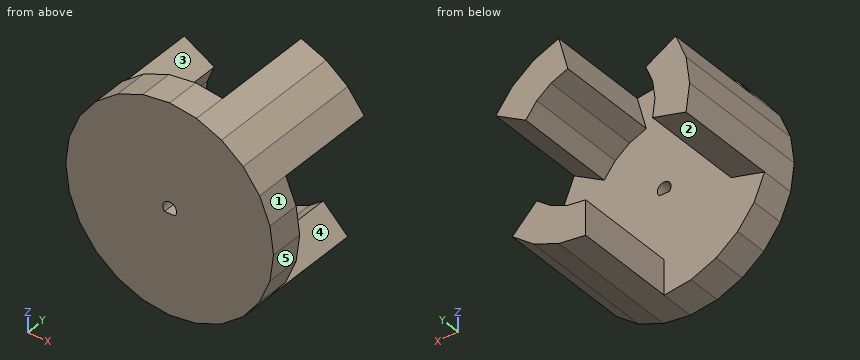
```python
from build123d import *

# Parameters (mm, degrees)
BOSS_EXTRUDE3_DEPTH   = 40
BOSS_EXTRUDE3_2_DEPTH = 40
BOSS_EXTRUDE3_3_DEPTH = 40
BOSS_EXTRUDE4_DEPTH   = 10


with BuildPart() as part:
    # Sketch1 → Boss-Extrude3 (new body)
    with BuildSketch(Plane(origin=(0, 0, 0), x_dir=(1, 0, 0), z_dir=(0, 1, 0))):
        Polygon((14.264167555, 14.264167555), (10.086289606, 17.469966057), (5.221047689, 19.485215243), (0, 20.172579212), (0, 30.258868817), (7.831571533, 29.227822865), (15.129434409, 26.204949086), (21.396251332, 21.396251332), align=None)
    extrude(amount=BOSS_EXTRUDE3_DEPTH)



with BuildPart() as body_2:
    # Sketch1 → Boss-Extrude3 2 (new body)
    with BuildSketch(Plane(origin=(0, 0, 0), x_dir=(1, 0, 0), z_dir=(0, 1, 0))):
        Polygon((5.221047689, -19.485215243), (10.086289606, -17.469966057), (14.264167555, -14.264167555), (17.469966057, -10.086289606), (26.204949086, -15.129434409), (21.396251332, -21.396251332), (15.129434409, -26.204949086), (7.831571533, -29.227822865), align=None)
    extrude(amount=BOSS_EXTRUDE3_2_DEPTH)


with BuildPart() as body_3:
    # Sketch1 → Boss-Extrude3 3 (new body)
    with BuildSketch(Plane(origin=(0, 0, 0), x_dir=(1, 0, 0), z_dir=(0, 1, 0))):
        Polygon((-19.485215243, 5.221047689), (-20.172579212, 0), (-19.485215243, -5.221047689), (-17.469966057, -10.086289606), (-26.204949086, -15.129434409), (-29.227822865, -7.831571533), (-30.258868817, 0), (-29.227822865, 7.831571533), align=None)
    extrude(amount=BOSS_EXTRUDE3_3_DEPTH)


with BuildPart() as part_1:
    add(part.part)

    add(body_2.part)  # Boss-Extrude4 merges body 2

    add(body_3.part)  # Boss-Extrude4 merges body 3
    # Sketch1_6 → Boss-Extrude4 (add)
    with BuildSketch(Plane(origin=(0, 0, 0), x_dir=(1, 0, 0), z_dir=(0, 1, 0))):
        Polygon((-29.227822865, 7.831571533), (-19.485215243, 5.221047689), (-20.172579212, 0), (-19.485215243, -5.221047689), (-17.469966057, -10.086289606), (-26.204949086, -15.129434409), (-21.396251332, -21.396251332), (-15.129434409, -26.204949086), (-7.831571533, -29.227822865), (0, -30.258868817), (7.831571533, -29.227822865), (5.221047689, -19.485215243), (10.086289606, -17.469966057), (14.264167555, -14.264167555), (17.469966057, -10.086289606), (26.204949086, -15.129434409), (29.227822865, -7.831571533), (30.258868817, 0), (29.227822865, 7.831571533), (26.204949086, 15.129434409), (21.396251332, 21.396251332), (14.264167555, 14.264167555), (10.086289606, 17.469966057), (5.221047689, 19.485215243), (0, 20.172579212), (0, 30.258868817), (-7.831571533, 29.227822865), (-15.129434409, 26.204949086), (-21.396251332, 21.396251332), (-26.204949086, 15.129434409), align=None)
        with BuildLine():
            Line((-1.5, 1.322875656), (1.5, 1.322875656))
            ThreePointArc((1.5, 1.322875656), (0, -2), (-1.5, 1.322875656))
        make_face(mode=Mode.SUBTRACT)
    extrude(amount=BOSS_EXTRUDE4_DEPTH)


solid = part_1.part
```
Input: part model. Units: mm. Frame: model coordinates. Face numbers are marked on the shaded views. A direction names the side the tool comes from. Give positions to 0.01 mm unless a question says otherwise; leave off trailing zeros. Order: outer loops, then holes, each group sorted by start corner. A loop starts at its lowest first (then second) coordinate and runs counter-clockwise, first axis right, second up. Notation, with made-up numbers: M -38,-7.5 L 10,-7.5 A14 ccw 10,6.5 Z; hole C 4.25,-19.75 d1. An arc over 180 degrees is marked long. Return JSON: item names as keys, results as strings.
1) Contact query for flat-ended pins moving along their axis: pin 1 (6 mm diameter, centred on x = 21.5, z = 6, fed in from +Y); pin 2 (4 mm diameter, centred on y = 28, z = -23, fed in from +X); pin 3 (5 mm diameter, centred on y = 18.5, z = 11, fed in from +X). Output: stop coordinate, or through.
Taken from the geometry:
{"pin 1": "stops at y = 10", "pin 2": "stops at x = 21.4", "pin 3": "stops at x = 23.38"}
2) Access query for the marked faces 1 and 2. Directions: +Z, -Z, +X, -X, +Y, -Y. A direction counts if a zero-diameter tool reaches every point of the face in a straight line with its end or side. Return the directions, or none.
Taken from the geometry:
{"face 1": "+Z, +X, +Y, -Y", "face 2": "-Z, +X, +Y"}
3) Section query D-D on z = 16. Output: boundary loops of the cut face in (x, y), and give its area (3 significant figures).
Taken from the geometry:
{"outline": "M -25.54,0 L 25.54,0 L 25.54,40 L 12,40 L 12,10 L -25.54,10 Z", "area": "917 mm2"}
4) Section query A-A on y = 22. Output: boundary loops of the cut face in (x, z), and give its area (3 significant figures).
Taken from the geometry:
{"outline": "M -30.26,0 L -29.23,-7.83 L -19.49,-5.22 L -20.17,0 L -19.49,5.22 L -17.47,10.09 L -26.2,15.13 L -29.23,7.83 Z; M 0,-30.26 L 7.83,-29.23 L 15.13,-26.2 L 21.4,-21.4 L 14.26,-14.26 L 10.09,-17.47 L 5.22,-19.49 L 0,-20.17 Z; M 5.22,19.49 L 10.09,17.47 L 14.26,14.26 L 17.47,10.09 L 26.2,15.13 L 21.4,21.4 L 15.13,26.2 L 7.83,29.23 Z", "area": "592 mm2"}
5) Mould query, pull axis Z, two halves, no side actions, for the marked faces 3, 4 and 5. Classes: released by +Z, released by -Z, zero draft, split by the parting line, or undercut.
Taken from the geometry:
{"face 3": "released by +Z", "face 4": "undercut", "face 5": "released by -Z"}
6) Line query: L1, parallel to Z at x = 0, y = 5; L2, parallel to X at y = 5, z = 0; L3, parallel to Y at x = -14.5, z = 20.5. Output: solid intervals per line, ascending. Write a range as [from, to].
Taken from the geometry:
{"L1": "z = [-30.26, -1.32], [2, 30.26]", "L2": "x = [-30.26, -2], [2, 30.26]", "L3": "y = [0, 10]"}
7) Section query C-C on x = 6. Output: boundary loops of the cut face in (y, z), and give its area (3 significant figures).
Taken from the geometry:
{"outline": "M 0,-29.47 L 40,-29.47 L 40,-19.16 L 10,-19.16 L 10,19.16 L 40,19.16 L 40,22.39 L 10,22.39 L 10,29.47 L 0,29.47 Z", "area": "995 mm2"}
8) Section query B-B on y = 9. Output: boundary loops of the cut face in (x, z), and give its area (3 significant figures).
Taken from the geometry:
{"outline": "M -30.26,0 L -29.23,-7.83 L -26.2,-15.13 L -21.4,-21.4 L -15.13,-26.2 L -7.83,-29.23 L 0,-30.26 L 7.83,-29.23 L 15.13,-26.2 L 21.4,-21.4 L 26.2,-15.13 L 29.23,-7.83 L 30.26,0 L 29.23,7.83 L 26.2,15.13 L 21.4,21.4 L 15.13,26.2 L 7.83,29.23 L 0,30.26 L -7.83,29.23 L -15.13,26.2 L -21.4,21.4 L -26.2,15.13 L -29.23,7.83 Z; hole M -1.5,-1.32 L 1.5,-1.32 A2 ccw long Z", "area": "2,830 mm2"}
